Answer from the drawing. Dimensions are ordinates in mm from the lowest x, y and z of the part. A direction names the side the tool comes from. Coordinates: 2 decimals unless noted, no trailing zeros. Write each loop counter-clockwise with the first axis right and the second up, starting at its lowest first coordinate (ties: lowest second). Pieces come first, ordered by that corner, then holes.
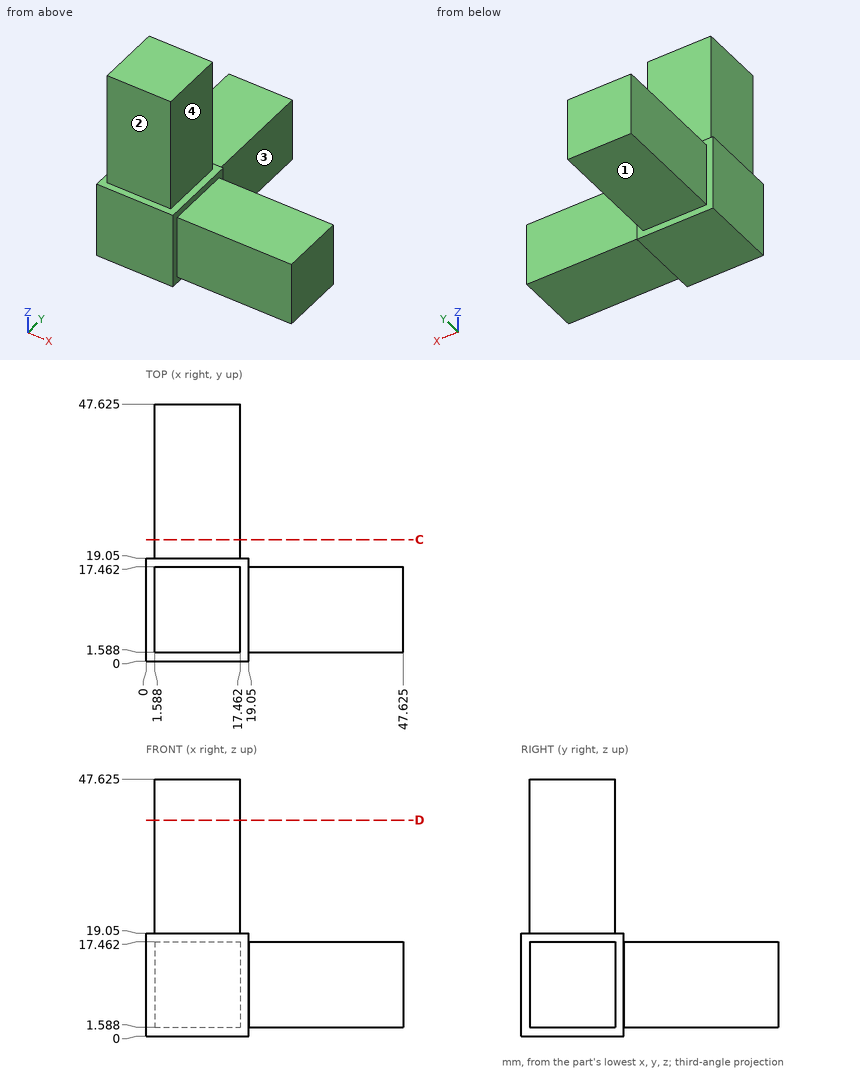
(1) Find the intervals of material crossed by probe 1 along Y at (x, z) = (13.5, 30), in increasing order.
(2) Section C-C, the plane y = 22.5 is taken. Write down the section's boundary in (x, z), plus the area to 3 significant figures.
(3) Which of the six approach directions +Z, -Z, +X, -X, +Y, -Y give full straight-line access (tool end or side, diameter ignored) to the marked faces 1, 2, 3 and 4?
(4) Each of these flat-tipped pins is pushed along its axis until it touches: pin 1 (12.5 mm diameter, centred on x = 7, y = 35, fed in from -Z); pin 2 (5 mm diameter, centred on y = 19.5, z = 38.5, fed in from +X); pin 3 (5 mm diameter, centred on y = 6.5, z = 31.5, fed in from -X). Where does it stop, or does it pass through?
Solution:
1. probe 1: y = 1.59 to 17.46
2. outline: (1.59, 1.59) - (17.46, 1.59) - (17.46, 17.46) - (1.59, 17.46) - close
2. area: 252 mm2
3. face 1: -Z, +X, -X, +Y
3. face 2: +Z, +X, -X, -Y
3. face 3: +Z, -Z, +X, +Y
3. face 4: +Z, +X, +Y, -Y
4. pin 1: stops at z = 1.59
4. pin 2: stops at x = 17.46
4. pin 3: stops at x = 1.59
